Build history of the part. All positions in model axes, mm. Face numbers are marked on the shaded views. A direction names the side the tool comes from. Round coordinates to 2 decimals unless told otherwise and drop trailing zeros. Loops run counter-clockwise (first coordinate to the right, second up) from the corner with the lowest first, then second, coordinate; pieces in that order, holes last. Notation, with made-up numbers: M 27.5,-26 L 39.5,-26 A23 cw 39.5,-18 Z; hole C 55.5,20 d11. An arc over 180 degrees is marked long. One line per item, written item: value.
```python
from build123d import *

# Parameters (mm, degrees)
SCHIZZO1_W                   = 30
SCHIZZO1_H                   = 20
SCHIZZO1_R                   = 7
ESTRUSIONE_ESTRUSIONE1_DEPTH = 4
SCHIZZO2_W                   = 4
SCHIZZO2_H                   = 20
ESTRUSIONE_ESTRUSIONE2_DEPTH = 30
SCHIZZO3_W                   = 8
SCHIZZO3_H                   = 20
ESTRUSIONE_ESTRUSIONE3_DEPTH = 3
SCHIZZO4_W                   = 8
SCHIZZO4_H                   = 20
ESTRUSIONE_ESTRUSIONE4_DEPTH = 3
RACCORDO1_R                  = 0.5
RACCORDO2_R                  = 0.5
RACCORDO3_R                  = 0.5
RACCORDO4_R                  = 0.5
RACCORDO5_R                  = 0.5
SCHIZZO5_R                   = 2.462201362
TAGLIO_ESTRUSIONE1_DEPTH     = 5


with BuildPart() as part:
    # Schizzo1 → Estrusione-Estrusione1 (new body)
    with BuildSketch(Plane.XY):
        with Locations((5, 0)):
            Rectangle(SCHIZZO1_W, SCHIZZO1_H)
        Circle(SCHIZZO1_R, mode=Mode.SUBTRACT)
    extrude(amount=ESTRUSIONE_ESTRUSIONE1_DEPTH)

    # Schizzo2 → Estrusione-Estrusione2 (add)
    with BuildSketch(Plane(origin=(0, 0, 0), x_dir=(-1, 0, 0), z_dir=(0, 0, -1))):
        with Locations((-22, 0)):
            Rectangle(SCHIZZO2_W, SCHIZZO2_H)
    extrude(amount=-ESTRUSIONE_ESTRUSIONE2_DEPTH)

    # Schizzo3 → Estrusione-Estrusione3 (add)
    with BuildSketch(Plane.XY.offset(30)):
        with Locations((24, 0)):
            Rectangle(SCHIZZO3_W, SCHIZZO3_H)
    extrude(amount=ESTRUSIONE_ESTRUSIONE3_DEPTH)

    # Schizzo4 → Estrusione-Estrusione4 (add)
    with BuildSketch(Plane(origin=(0, 0, 0), x_dir=(-1, 0, 0), z_dir=(0, 0, -1))):
        with Locations((-24, 0)):
            Rectangle(SCHIZZO4_W, SCHIZZO4_H)
    extrude(amount=ESTRUSIONE_ESTRUSIONE4_DEPTH)

    # Raccordo1
    raccordo1_edges = [part.edges().sort_by_distance(p)[0] for p in [
        (20, 0, 4),
        (24, 0, 30),
        (24, 0, 0),
        (20, 0, 0),
    ]]
    fillet(raccordo1_edges, radius=RACCORDO1_R)

    # Raccordo2
    raccordo2_edges = [part.edges().sort_by_distance(p)[0] for p in [
        (4.75, -10, 0),
        (20, -10, -1.75),
        (4.75, 10, 0),
        (19.853553391, 10, -0.146446609),
        (19.853553391, -10, -0.146446609),
        (28, 0, 0),
        (20, 10, -1.75),
    ]]
    fillet(raccordo2_edges, radius=RACCORDO2_R)

    # Raccordo3
    raccordo3_edges = [part.edges().sort_by_distance(p)[0] for p in [
        (26.25, -10, 30),
        (24, -10, 15),
        (28, -10, -1.75),
        (27.853553391, -10, -0.146446609),
        (24.146446609, -10, 29.853553391),
        (24.146446609, -10, 0.146446609),
        (26, -10, 0),
    ]]
    fillet(raccordo3_edges, radius=RACCORDO3_R)

    # Raccordo4
    raccordo4_edges = [part.edges().sort_by_distance(p)[0] for p in [
        (28, 0.25, 30),
        (28, -9.853553391, 30.146446609),
        (28, -10, 31.75),
        (26.25, 10, 30),
        (24, 10, 15),
        (28, 10, -1.75),
        (27.853553391, 10, -0.146446609),
        (24.146446609, 10, 29.853553391),
        (24.146446609, 10, 0.146446609),
        (26, 10, 0),
    ]]
    fillet(raccordo4_edges, radius=RACCORDO4_R)

    # Raccordo5
    raccordo5_edges = [part.edges().sort_by_distance(p)[0] for p in [
        (20, 0, -3),
        (20.146446609, -9.853553391, -3),
        (20.146446609, 9.853553391, -3),
        (24, -10, -3),
        (27.853553391, -9.853553391, -3),
        (28, 0.25, 33),
        (28, 0, -3),
        (27.853553391, 9.853553391, -3),
        (27.853553391, -9.853553391, 33),
        (20, 10, 18.75),
        (20, -10, 18.75),
        (20, 0, 33),
        (23.75, -10, 33),
        (24, 10, 33),
        (-10, 0, 4),
        (4.75, 10, 4),
        (19.853553391, 10, 4.146446609),
        (19.853553391, -10, 4.146446609),
        (-10, 10, 2.25),
        (-10, -10, 2.25),
        (4.75, -10, 4),
        (24, 10, -3),
        (-10, 0, 0),
        (-10, -9.853553391, 0.146446609),
        (-10, 9.853553391, 0.146446609),
    ]]
    fillet(raccordo5_edges, radius=RACCORDO5_R)

    # Schizzo5 → Taglio-Estrusione1 (cut)
    with BuildSketch(Plane(origin=(24, 0, 0), x_dir=(0, 0, -1), z_dir=(1, 0, 0))):
        with Locations((-15, 0)):
            Circle(SCHIZZO5_R)
    extrude(amount=-TAGLIO_ESTRUSIONE1_DEPTH, mode=Mode.SUBTRACT)


solid = part.part
```
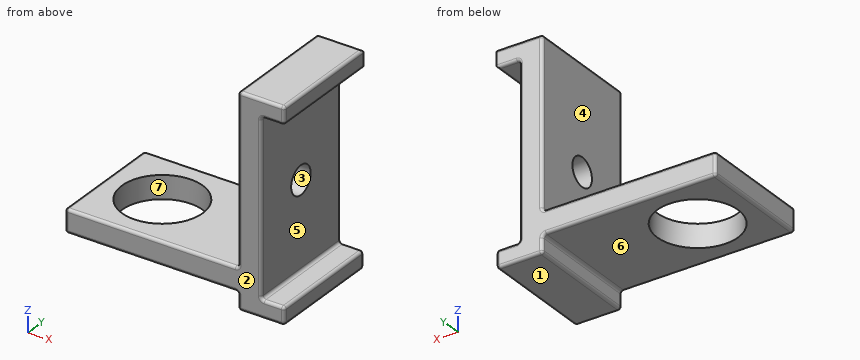
Item 1: Slice it at B-B, the plane x = 0. Give the cut face in (y, z), and give its area (3 significant figures).
Check values:
outline: M -10,0.5 A0.5 ccw -9.5,0 L -7,0 L -7,4 L -9.5,4 A0.5 ccw -10,3.5 Z; M 7,0 L 9.5,0 A0.5 ccw 10,0.5 L 10,3.5 A0.5 ccw 9.5,4 L 7,4 Z
area: 23.8 mm2
Item 2: Wall check: line 1 along Y through (x, z) = (22.3, 15); line 2 along Z through (x, y) = (16, -4.5); line 3 along Y through (x, z) = (0, 1.35). Give the ranges that are in metal, low to high.
Check values:
line 1: y = -10 to -2.46, 2.46 to 10
line 2: z = 0 to 4
line 3: y = -10 to -7, 7 to 10
Item 3: Slice it at D-D, the plane y = -6.25. Give the cut face in (x, z).
Check values:
outline: M -10,0.5 A0.5 ccw -9.5,0 L -3.15,0 L -3.15,4 L -9.5,4 A0.5 ccw -10,3.5 Z; M 3.15,0 L 19.5,0 A0.5 cw 20,-0.5 L 20,-2.5 A0.5 ccw 20.5,-3 L 27.5,-3 A0.5 ccw 28,-2.5 L 28,-0.5 A0.5 ccw 27.5,0 L 24.5,0 A0.5 cw 24,0.5 L 24,29.5 A0.5 cw 24.5,30 L 27.5,30 A0.5 ccw 28,30.5 L 28,32.5 A0.5 ccw 27.5,33 L 20.5,33 A0.5 ccw 20,32.5 L 20,4.5 A0.5 cw 19.5,4 L 3.15,4 Z
Item 4: Slice it at C-C, the plane z = 15. Give the cut face in (x, y).
Check values:
outline: M 20,-9.5 A0.5 ccw 20.5,-10 L 23.5,-10 A0.5 ccw 24,-9.5 L 24,-2.46 L 20,-2.46 Z; M 20,2.46 L 24,2.46 L 24,9.5 A0.5 ccw 23.5,10 L 20.5,10 A0.5 ccw 20,9.5 Z
Item 5: Pull direction Y, two halves, no side cores. Call the marked faces 1, 2 and 3: pulls with the +Y half, pulls with the -Y half, needs draft (parallel to the pull), parting line crosses it, or undercut.
Check values:
face 1: needs draft
face 2: pulls with the -Y half
face 3: undercut
Item 6: Drop flat-ended pins along their axis: P1, Ø9.5, axis at x = 10, y = 0.5, coming from the -Z side; P2, Ø1, axis at y = 3.5, z = -1, coming from the -X side; P3, Ø5.5, axis at x = 9.5, y = 3.5, coming from the +Z side. Give the stop position or say it passes through.
Check values:
P1: stops at z = 0
P2: stops at x = 20
P3: stops at z = 4
Item 7: Which spindle directions (+Z, -Z, +X, -X, +Y, -Y) get a long thin tool onto all of the face, cutting with end or side? Do the marked faces 4, 5, 6 and 7. Say none if no direction does.
Check values:
face 4: +Z, -X, +Y, -Y
face 5: +X, +Y, -Y
face 6: -Z, -X, +Y, -Y
face 7: +Z, -Z
Item 8: Slice it at A-A, the plane y = 0. Give the number of separate pieces and of enclosed holes in the cut face, and give its area (3 significant figures).
Check values:
separate pieces: 3
enclosed holes: 0
area: 212 mm2
